Verification items for this drawing (mm, ordinates from the low corner). A direction names the side the tool comes from. Round coordinates to 2 decimals unless told otherwise and drop trailing zeros. Order: outer loops, then holes, each group sorted by start corner. A loop starts at its lowest first (then second) coordinate and runs counter-clockwise, first axis right, second up. Notation, with made-up numbers: (66, -10) -> (86, -10) arc R15 cw to (86, -6) -> close; hole circle Ø8 at (55.5, -11.5). An arc over 180 degrees is marked (long way). Answer in a Markdown table with one row per item. Add a question column.
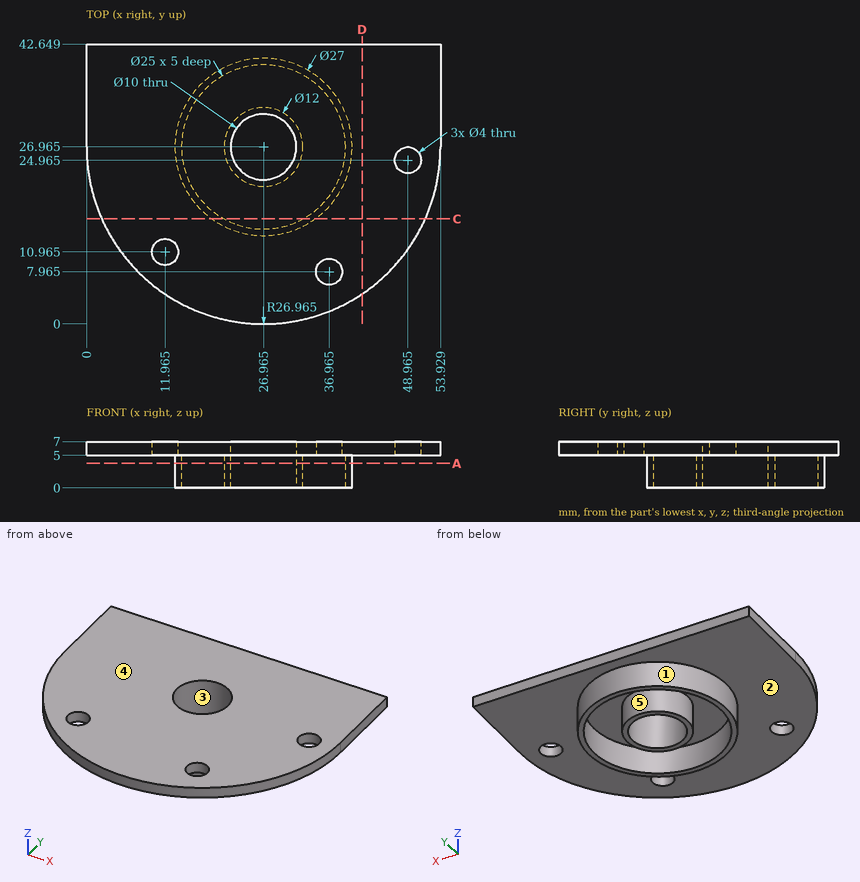
1) Cross-section at D-D, the plane x = 42. Record the boundary of the cut face in (y, z).
2) Depth check by flat-ended pin: P1, Ø5, axis at x = 31, y = 19, coming from the -Z side; P2, Ø1.5, axis at x = 37, z = 6, coming from the -Y side; P3, Ø4, axis at x = 34.5, z = 3.5, coming from the -Y side (1 decimal). Enter the tip coordinate at first touch or a pass-through.
3) Cross-section at A-A, the plane z = 3.75. Record the boundary of the cut face in (x, y) (1 decimal).
4) Draft check along Y on the marked faces 1, 2 and 3. Enter one of: +Y half, -Y half, draft (parallel to the pull), parting line (faces both ways), or undercut.
5) Tool access check on the marked faces 4 and 5. Record the directions out of +Z, -Z, +X, -X, +Y, -Y that give a thin tool (end or side, any length) a straight path to the whole face; none if there is none.
6) Cross-section at C-C, the plane y = 16. Record the boundary of the cut face in (x, z).
7) Thickness scan on L1, parallel to Z at x = 12.5, y = 20.5; L2, parallel to X at y = 35, z = 4 (1 decimal); L3, parallel to Y at x = 30, z = 4. Record the ranges inside material, lowest first. Write a range as [from, to].
Results below:
| question | item | result |
|---|---|---|
| 1 | outline | (4.58, 5) -> (42.65, 5) -> (42.65, 7) -> (4.58, 7) -> close |
| 2 | P1 | z = 5 |
| 2 | P2 | y = 1.65 |
| 2 | P3 | y = 0.7 |
| 3 | outline | circle Ø27 at (27, 27); circle Ø12 at (27, 27); hole circle Ø25 at (27, 27); hole circle Ø10 at (27, 27) |
| 4 | face 1 | parting line |
| 4 | face 2 | draft |
| 4 | face 3 | undercut |
| 5 | face 4 | +Z, +X, -X, +Y, -Y |
| 5 | face 5 | -Z |
| 6 | outline | (2.33, 5) -> (19.09, 5) -> (19.09, 0) -> (20.96, 0) -> (20.96, 5) -> (32.97, 5) -> (32.97, 0) -> (34.84, 0) -> (34.84, 5) -> (51.6, 5) -> (51.6, 7) -> (2.33, 7) -> close |
| 7 | L1 | [5, 7] |
| 7 | L2 | [16.1, 17.4], [36.5, 37.8] |
| 7 | L3 | [13.81, 14.84], [21.79, 22.99], [30.94, 32.14], [39.09, 40.12] |
